Autodesk Inventor part; units mm, degrees
ref_plane "YZ Plane" through (0, 0, 0) normal (1, 0, 0) x (0, 1, 0)
ref_plane "XZ Plane" through (0, 0, 0) normal (0, 1, 0) x (-1, 0, 0)
ref_plane "XY Plane" through (0, 0, 0) normal (0, 0, 1) x (1, 0, 0)
sketch "Sketch1" plane through (0, 0, 0) normal (0, 1, 0) x (-1, 0, 0)
  line L0 (480.5, 0) -> (480.5, -30)
  arc A0 (445.9689, -77.547) -> (480.5, -30) centre (430.5, -30) ccw
  arc A1 (0, -148.2683) -> (445.9689, -77.547) centre (0, 1293.2317) ccw
  line L1 (0, 191.6842) -> (0, -191.6842)
  arc A2 (0, -142.2683) -> (444.1126, -71.8413) centre (0, 1293.2317) ccw
  arc A3 (444.1126, -71.8413) -> (474.5, -30) centre (430.5, -30) ccw
  line L2 (474.5, -30) -> (474.5, 0)
  line L3 (474.5, 0) -> (480.5, 0)
  line L4 (0, -142.2683) -> (0, -148.2683)
  point P0 (0, 0)
  point P1 (0, 0)
  point P2 (0, -145.2683)
  dimension "d0" = 50
  dimension "d1" = 30
  dimension "d3" = 1441.5
  dimension "d4" = 480.5
  dimension "d6" = 6
revolve "Revolution1" add sketch "Sketch1" angle 360 about axis through (0, 0, 191.6842) along (0, 0, -1)
sketch "Sketch2" plane through (0, 0, 0) normal (0, 0, 1) x (1, 0, 0)
  circle A0 centre (0, 0) radius 16.75
  dimension "d8" = 33.5
extrude "Extrusion1" cut sketch "Sketch2" against normal through all
properties part number "Сферическое дно D1000"
Geometry check sheet. Reference: the model listing, model coordinates, mm. Round coordinates to 2 decimals unless told otherwise and drop trailing zeros. Use a Markdown table: item, result.
(1) Mould release check, pull along X, two halves, no side actions. Record for faces 1 (the flat face through (-354, -318, 0)), 2 (the cylindrical face through (104.163, -469.074, -15.21)), 3 (the cylindrical face through (474.04, -20.86, -14.79)): released by +X, released by -X, zero draft, split by the parting line, or undercut.
Calculated:
| item | result |
|---|---|
| face 1 | zero draft |
| face 2 | split by the parting line |
| face 3 | undercut |
(2) Scan lines: probe 1 along Y at (x, z) = (0, -11); probe 2 along X at (y, z) = (408.5, -45); probe 3 along Y at (x, z) = (-300, -50). Record each from-to range of solid material in increasing order.
Calculated:
| item | result |
|---|---|
| probe 1 | -480.5 to -474.5, 474.5 to 480.5 |
| probe 2 | -248.6 to -236.19, 236.19 to 248.6 |
| probe 3 | -369.98 to -361.4, 361.4 to 369.98 |
(3) Go/stop test with flat-tipped pins: P1, Ø5, axis at x = 179.5, z = -17, coming from the +Y side; P2, Ø12, axis at x = -354, y = 45, coming from the +Z side; P3, Ø4, axis at x = -21, y = 285, coming from the +Z side. Record where each tip stops, or that it passes through.
Calculated:
| item | result |
|---|---|
| P1 | y = 446.71 |
| P2 | z = -95.65 |
| P3 | z = -113.13 |
